Model file for the job. Use its own axes, mm. Give positions to 0.01 mm unless a question says otherwise; leave off trailing zeros. Order: outer loops, then holes, each group sorted by start corner. A loop starts at its lowest first (then second) coordinate and runs counter-clockwise, first axis right, second up. Notation, with made-up numbers: M -19,-22 L -10,-22 A15 ccw -10,-18 Z; hole C -27.5,33.25 d4. An arc over 180 degrees is marked long. Return JSON: item names as keys, results as strings. Group by question number.
1. Slice it at B-B on x = -4. List the corners of the cut face in (y, z), then the cut area to 3 significant figures.
2. Slice it at A-A on z = 0.7. List the corners of the cut face in (x, y).
3. Slice it at C-C on x = 11.5. List the corners of the cut face in (y, z).
4. Wall check: probe 1 along Y at (x, z) = (-15.5, 0.5); probe 2 along Y at (x, z) = (-4, 0.7); probe 3 along Y at (x, z) = (15, 0.4). Give the ranges that are in metal, low to high. Write a range as [from, to].
from build123d import *

# Parameters (mm, degrees)
CROQUIS1_R              = 1.5
CROQUIS1_R_2            = 2
SALIENTE_EXTRUIR1_DEPTH = 1.5


with BuildPart() as part:
    # Croquis1 → Saliente-Extruir1 (new body)
    with BuildSketch(Plane.XY):
        with BuildLine():
            Line((0, 0), (-16, 0))
            ThreePointArc((-16, 0), (-17.414213562, 0.585786438), (-18, 2))
            Line((-18, 2), (-18, 34))
            ThreePointArc((-18, 34), (-17.414213562, 35.414213562), (-16, 36))
            Line((-16, 36), (-10.5, 36))
            ThreePointArc((-10.5, 36), (-9.085786438, 36.585786438), (-8.5, 38))
            Line((-8.5, 38), (-8.5, 50))
            ThreePointArc((-8.5, 50), (-7.914213562, 51.414213562), (-6.5, 52))
            Line((-6.5, 52), (0, 52))
            Line((0, 52), (6.5, 52))
            ThreePointArc((6.5, 52), (7.914213562, 51.414213562), (8.5, 50))
            Line((8.5, 50), (8.5, 38))
            ThreePointArc((8.5, 38), (9.085786438, 36.585786438), (10.5, 36))
            Line((10.5, 36), (16, 36))
            ThreePointArc((16, 36), (17.414213562, 35.414213562), (18, 34))
            Line((18, 34), (18, 2))
            ThreePointArc((18, 2), (17.414213562, 0.585786438), (16, 0))
            Line((16, 0), (0, 0))
        make_face()
        with Locations((-15.5, 2.5)):
            Circle(CROQUIS1_R, mode=Mode.SUBTRACT)
        with Locations((-15.5, 33.5)):
            Circle(CROQUIS1_R, mode=Mode.SUBTRACT)
        with Locations((-4, 47.5)):
            Circle(CROQUIS1_R_2, mode=Mode.SUBTRACT)
        with Locations(Location((4, 47.5, 0), (0, 0, 180))):
            Circle(CROQUIS1_R_2, mode=Mode.SUBTRACT)
        with Locations(Location((15.5, 33.5, 0), (0, 0, 180))):
            Circle(CROQUIS1_R, mode=Mode.SUBTRACT)
        with Locations(Location((15.5, 2.5, 0), (0, 0, 180))):
            Circle(CROQUIS1_R, mode=Mode.SUBTRACT)
    extrude(amount=SALIENTE_EXTRUIR1_DEPTH)


solid = part.part
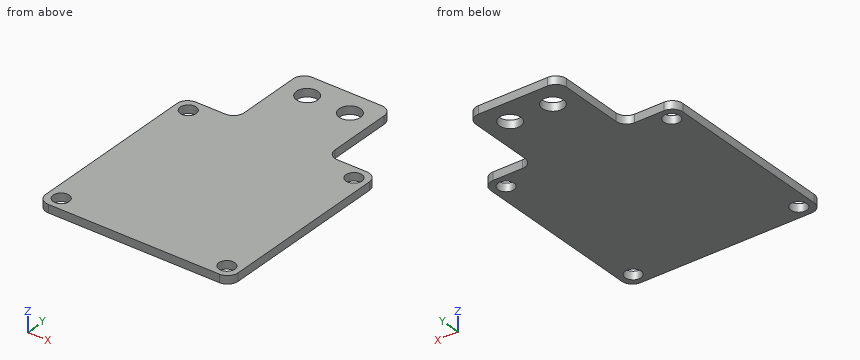
Result:
{
 "1": {"outline": "M 0,0 L 45.5,0 L 45.5,1.5 L 0,1.5 Z; M 49.5,0 L 52,0 L 52,1.5 L 49.5,1.5 Z", "area": "72.0 mm2"},
 "2": {"outline": "M -18,2 A2 ccw -16,0 L 16,0 A2 ccw 18,2 L 18,34 A2 ccw 16,36 L 10.5,36 A2 cw 8.5,38 L 8.5,50 A2 ccw 6.5,52 L -6.5,52 A2 ccw -8.5,50 L -8.5,38 A2 cw -10.5,36 L -16,36 A2 ccw -18,34 Z; hole C -15.5,2.5 d3; hole C -15.5,33.5 d3; hole C -4,47.5 d4; hole C 4,47.5 d4; hole C 15.5,2.5 d3; hole C 15.5,33.5 d3"},
 "3": {"outline": "M 0,0 L 36,0 L 36,1.5 L 0,1.5 Z"},
 "4": {"probe 1": "y = [0, 1], [4, 32], [35, 36]", "probe 2": "y = [0, 45.5], [49.5, 52]", "probe 3": "y = [0, 1.09], [3.91, 32.09], [34.91, 36]"}
}
